from build123d import *

# Parameters (mm, degrees)
RESSALTO_EXTRUS_O1_DEPTH = 5
ESBO_O2_R                = 1.5
CORTE_EXTRUS_O1_DEPTH    = 5
FILETE1_R                = 10


with BuildPart() as part:
    # Esboço1 → Ressalto-extrusão1 (new body)
    with BuildSketch(Plane.XY):
        with BuildLine():
            Line((-14.089663978, 13.135393664), (-14.089663978, 28.135393664))
            Line((-14.089663978, 28.135393664), (-34.089663978, 28.135393664))
            Line((-34.089663978, 28.135393664), (-34.089663978, 158.135393664))
            Line((-34.089663978, 158.135393664), (25.910336022, 158.135393664))
            Line((25.910336022, 158.135393664), (25.910336022, 28.135393664))
            Line((25.910336022, 28.135393664), (5.910336022, 28.135393664))
            Line((5.910336022, 28.135393664), (5.910336022, 13.135393664))
            ThreePointArc((5.910336022, 13.135393664), (-4.089663978, 3.135393664), (-14.089663978, 13.135393664))
        make_face()
    extrude(amount=RESSALTO_EXTRUS_O1_DEPTH)

    # Esboço2 → Corte-extrusão1 (cut)
    with BuildSketch(Plane.XY.offset(5)):
        with Locations((-4.089663978, 13.135393664)):
            Circle(ESBO_O2_R)
    extrude(amount=-CORTE_EXTRUS_O1_DEPTH, mode=Mode.SUBTRACT)

    # Filete1
    filete1_edges = [part.edges().sort_by_distance(p)[0] for p in [
        (-14.089663978, 28.135393664, 2.5),
    ]]
    fillet(filete1_edges, radius=FILETE1_R)
    filete1_2_edges = [part.edges().sort_by_distance(p)[0] for p in [
        (-34.089663978, 28.135393664, 2.5),
    ]]
    fillet(filete1_2_edges, radius=FILETE1_R - 0.0001)  # a hair under: the kernel refuses the full size
    filete1_3_edges = [part.edges().sort_by_distance(p)[0] for p in [
        (5.910336022, 28.135393664, 2.5),
    ]]
    fillet(filete1_3_edges, radius=FILETE1_R)
    filete1_4_edges = [part.edges().sort_by_distance(p)[0] for p in [
        (25.910336022, 28.135393664, 2.5),
    ]]
    fillet(filete1_4_edges, radius=FILETE1_R - 0.0001)  # a hair under: the kernel refuses the full size


solid = part.part
Could you check a few things on this model? Use its own coordinates, in mm. A direction names the side the tool comes from. Give positions to 0.01 mm unless a question says otherwise; leave off trailing zeros. Order: outer loops, then holes, each group sorted by start corner. A loop starts at its lowest first (then second) coordinate and runs counter-clockwise, first axis right, second up. Notation, with made-up numbers: (-10.5, 77) - (38.5, 77) arc R27 ccw to (38.5, 100) - close; hole circle Ø11 at (-21.5, -7). An arc over 180 degrees is marked (long way). One line per question, with ' | ' between items. Start each with the question number.
Item 1: For faces 5 (the flat face through (5.91, 16, 2)), 6 (the flat face through (-14.09, 16, 2)), 7 (the flat face through (-34.09, 97, 2)), which set-ups out of +Z, -Z, +X, -X, +Y, -Y let a thin tool reach every point of the face, with its end or its side?
Item 2: Thinking about a two-plate mould opening in Y: for faces 1 (the cylindrical face through (-4.41, 11.67, 2.54)), 2 (the cylindrical face through (-31.083, 30.987, 2.535)), 3 (the flat face through (-5, 158.135, 2)), 4 (the flat face through (-4, 82, 0)), which applies, pulls with the +Y half, pulls with the -Y half, needs draft (parallel to the pull), parting line crosses it, or undercut?
Item 3: I'm going to push flat-ended pins straight in: pin 1 Ø2.5 at (y, z) = (15, 2.5) entering from +X; pin 2 Ø6 at (x, y) = (12.5, 89) entering from -Z; pin 3 Ø1.5 at (y, z) = (14.5, 1.5) entering from -X. Where does each tip first touch, or does it pass through?
Item 4: I want a section at B-B on x = -16.5. Write out the boundary of the cut face in (y, z), then the cut area to 3 significant figures.
Item 5: I want a section at C-C on x = 12. Write out the boundary of the cut face in (y, z), then the cut area to 3 significant figures.
Item 6: I need wall thicknesses on probe 1 along X at (y, z) = (15.5, 4.4); probe 2 along X at (y, z) = (12.5, 1.9); probe 3 along Y at (x, z) = (15, 1.2). Which ranges of each line are inside material? Lowest first, please. Write a range as [from, to].
Verdict:
1) face 5: +Z, -Z, +X, -Y | face 6: +Z, -Z, -X, -Y | face 7: +Z, -Z, -X, +Y, -Y
2) face 1: undercut | face 2: pulls with the -Y half | face 3: pulls with the +Y half | face 4: needs draft
3) pin 1: x = 5.91 | pin 2: z = 0 | pin 3: x = -14.09
4) outline: (24.65, 0) - (158.14, 0) - (158.14, 5) - (24.65, 5) - close | area: 667 mm^2
5) outline: (27.34, 0) - (158.14, 0) - (158.14, 5) - (27.34, 5) - close | area: 654 mm^2
6) probe 1: [-14.09, 5.91] | probe 2: [-14.07, -5.45], [-2.73, 5.89] | probe 3: [28.09, 158.14]
